For this review, take the finished solid that the model builds, in its own axes (mm). A direction names the side the tool comes from. Coordinates: 2 decimals unless noted, no trailing zeros. Loops run counter-clockwise (first coordinate to the right, second up) from the corner with the lowest first, then second, coordinate; pieces in that order, holes last. Notation, with made-up numbers: M 70.5,-21.5 L 118.5,-21.5 A6 ccw 118.5,-15.5 Z; hole C 49.5,-17 d2. An arc over 180 degrees is marked long. Write each question's results on one line, items separated by ' | '. Start each with the question number.
```python
from build123d import *

# Parameters (mm, degrees)
SKETCH1_R           = 2.508000064
BASE_FLANGE1_DEPTH  = 3.175
BOSS_EXTRUDE1_DEPTH = 3.175
SKETCH10_W          = 73.528573301
SKETCH10_H          = 32.63252049
CUT_EXTRUDE1_DEPTH  = 148.382240559


# Sheet-metal steps are written as plain solids
with BuildPart() as part:
    # Sketch1 → Base-Flange1 (new body)
    with BuildSketch(Plane.XY):
        Polygon((-8.910000095, 75.81), (21.268467492, 75.81), (73.931530887, 75.81), (104.109998474, 75.81), (104.109998474, -7.01), (73.931530887, -7.01), (73.931530887, 50.41), (21.268467492, 50.41), (21.268467492, -7.01), (-8.910000095, -7.01), align=None)
        with Locations((-2.560000095, 56.76)):
            Circle(SKETCH1_R, mode=Mode.SUBTRACT)
        with Locations((11.409999905, -0.66)):
            Circle(SKETCH1_R, mode=Mode.SUBTRACT)
        with Locations(Location((83.789998474, -0.66, 0), (0, 0, 180))):
            Circle(SKETCH1_R, mode=Mode.SUBTRACT)
        with Locations(Location((97.759998474, 56.76, 0), (0, 0, 180))):
            Circle(SKETCH1_R, mode=Mode.SUBTRACT)
    extrude(amount=-BASE_FLANGE1_DEPTH)

    # Sketch9 → Boss-Extrude1 (add)
    with BuildSketch(Plane(origin=(0, 75.81, 0), x_dir=(1, 0, 0), z_dir=(0, 1, 0))):
        Polygon((-8.910000095, 3.175), (-8.910000095, 59.055), (104.109998474, 59.055), (104.109998474, 0), (-8.910000095, 0), align=None)
    extrude(amount=BOSS_EXTRUDE1_DEPTH)

    # Sketch10 → Cut-Extrude1 (cut, through all)
    with BuildSketch(Plane(origin=(0, 78.985, 0), x_dir=(1, 0, 0), z_dir=(0, 1, 0))):
        with Locations((47.59999919, 29.5275)):
            Rectangle(SKETCH10_W, SKETCH10_H)
    extrude(amount=-CUT_EXTRUDE1_DEPTH, mode=Mode.SUBTRACT)


solid = part.part
```
Q1. Take a section at B-B, the plane x = -2.56. Give the boundary of the cut face in (y, z) (3 decimals), then the cut area to 3 significant figures.
Q2. Insertion check: P1, Ø4, axis at x = -2.56, y = 56.76, coming from the -Z side; P2, Ø1, axis at x = 46.5, y = 59, coming from the -Z side (3 decimals); P3, Ø1, axis at x = 48.5, z = -2.5, coming from the -Y side. Each pin has a flat end and moves straight along its axis. Give the tip position at first contact, or say it passes through.
Q3. The part is to be moulded in two halves that separate along Z. For faces 5 (the face through (47, 77, -45.844)), 6 (the face through (47, 77, -59.055)), 7 (the face through (-8.91, 55, -1)), say which applies: pulls with the +Z half, pulls with the -Z half, needs draft (parallel to the pull), parting line crosses it, or undercut.
Q4. Take a section at C-C, the plane z = -34.5. Give the boundary of the cut face in (x, y) (3 decimals), then the cut area to 3 significant figures.
Q5. Take a section at D-D, the plane y = 9.5. Give the boundary of the cut face in (x, z) (3 decimals), then the cut area to 3 significant figures.
Q6. For faces 1 (the face through (48, 50.41, -2)), 2 (the face through (47, 77, -13.211)), 3 (the face through (48, 75.81, -50)), 4 (the face through (104.11, 55, -1)), list the 3-axis set-ups (+Z, -Z, +X, -X, +Y, -Y) from which the entire face can be reached by the end or side of a thin tool; tool diameter is ignored.
Q7. Take a section at A-A, the plane y = 56.76. Give the boundary of the cut face in (x, z) (3 decimals), then the cut area to 3 significant figures.
Q8. To check wall thickness, follow line 1 along Y through (x, z) = (11.41, -1.7) (3 decimals); line 2 along Z through (x, y) = (9, -1.5) (3 decimals); line 3 along Y through (x, z) = (31, -11) (3 decimals). State the ranges of each line that lie inside material, in increasing order.
Results:
1) outline: M -7.01,-3.175 L 54.252,-3.175 L 54.252,0 L -7.01,0 Z; M 59.268,-3.175 L 75.81,-3.175 L 75.81,-59.055 L 78.985,-59.055 L 78.985,0 L 59.268,0 Z | area: 435 mm^2
2) P1: through | P2: z = -3.175 | P3: y = 50.41
3) face 5: undercut | face 6: pulls with the -Z half | face 7: needs draft
4) outline: M -8.91,75.81 L 10.836,75.81 L 10.836,78.985 L -8.91,78.985 Z; M 84.364,75.81 L 104.11,75.81 L 104.11,78.985 L 84.364,78.985 Z | area: 125 mm^2
5) outline: M -8.91,-3.175 L 21.268,-3.175 L 21.268,0 L -8.91,0 Z; M 73.932,-3.175 L 104.11,-3.175 L 104.11,0 L 73.932,0 Z | area: 192 mm^2
6) face 1: +Z, -Z, -Y | face 2: +Y, -Y | face 3: -Z, +X, -X, -Y | face 4: +Z, -Z, +X, +Y, -Y
7) outline: M -8.91,-3.175 L -5.068,-3.175 L -5.068,0 L -8.91,0 Z; M -0.052,-3.175 L 95.252,-3.175 L 95.252,0 L -0.052,0 Z; M 100.268,-3.175 L 104.11,-3.175 L 104.11,0 L 100.268,0 Z | area: 327 mm^2
8) line 1: -7.01 to -3.168, 1.848 to 78.985 | line 2: -3.175 to 0 | line 3: 75.81 to 78.985
